The drawing under review shows one solid part. Ordinate dimensions are in mm from its lowest x, y, z. Give positions to 0.01 mm unless a question says otherwise; leave off trailing zeros. Order: outer loops, then holes, each group sorted by start corner. A loop starts at its lowest first (then second) coordinate and runs counter-clockwise, first axis right, second up. Notation, with made-up numbers: (-28, -10) -> (10, -10) arc R13 cw to (10, 8) -> close; hole circle Ø4 at (-25.5, -22). An arc over 180 degrees is marked (long way). Use a Markdown table: item, result. Add a question column.
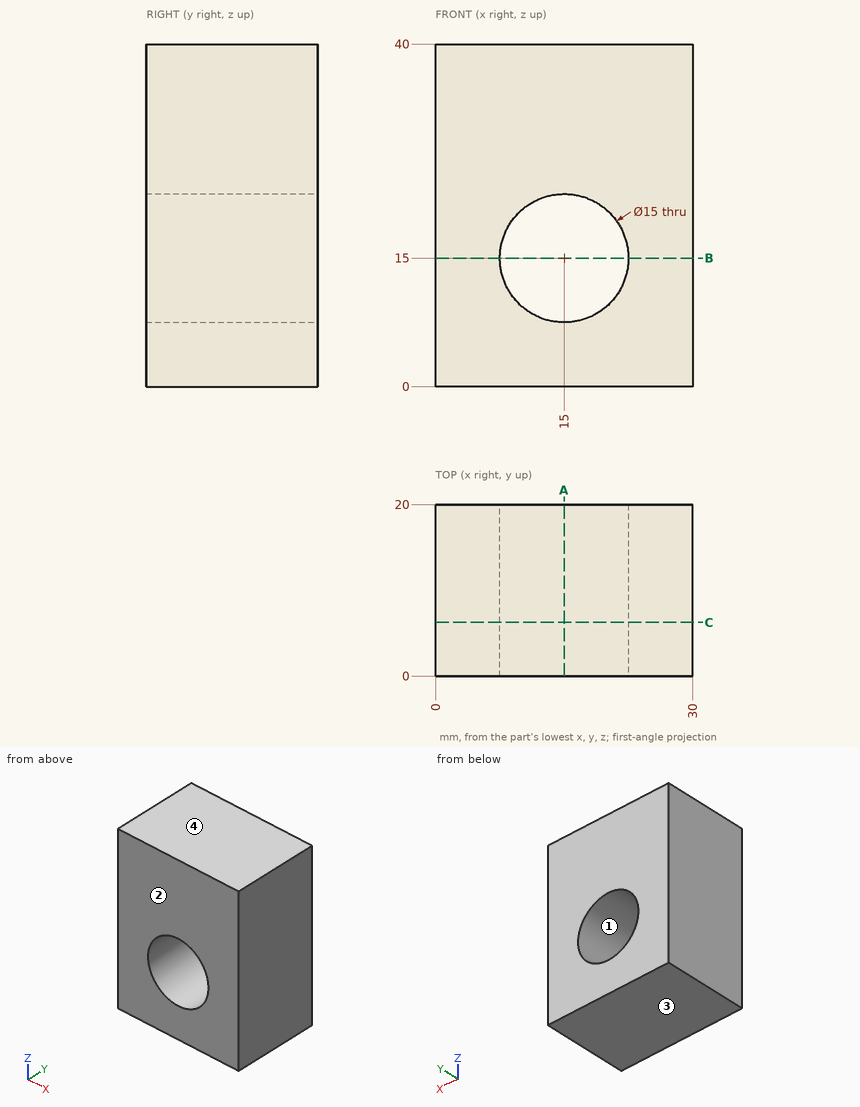
1) For L1, parallel to Z at x = 15, y = 14.5; L2, parallel to X at y = 4.75, z = 15; L3, parallel to Z at x = 16.5, y = 12.5, list the stretches that pass through material, from the lowest coordinate up. Write a range as [from, to].
2) The part is to be moulded in two halves that separate along Z. For the marked faces 1, 2, 3 and 4, say which applies: +Z half, -Z half, draft (parallel to the pull), parting line (faces both ways), or undercut.
3) Add section B-B (z = 15). Give the boundary of the cut face in (x, y).
4) Add section A-A (x = 15). Give the boundary of the cut face in (y, z).
5) Add section C-C (y = 6.25). Give the boundary of the cut face in (x, z), then the cut area to 3 significant figures.
Worked answers:
| question | item | result |
|---|---|---|
| 1 | L1 | [0, 7.5], [22.5, 40] |
| 1 | L2 | [0, 7.5], [22.5, 30] |
| 1 | L3 | [0, 7.65], [22.35, 40] |
| 2 | face 1 | undercut |
| 2 | face 2 | draft |
| 2 | face 3 | -Z half |
| 2 | face 4 | +Z half |
| 3 | outline | (0, 0) -> (7.5, 0) -> (7.5, 20) -> (0, 20) -> close; (22.5, 0) -> (30, 0) -> (30, 20) -> (22.5, 20) -> close |
| 4 | outline | (0, 0) -> (20, 0) -> (20, 7.5) -> (0, 7.5) -> close; (0, 22.5) -> (20, 22.5) -> (20, 40) -> (0, 40) -> close |
| 5 | outline | (0, 0) -> (30, 0) -> (30, 40) -> (0, 40) -> close; hole circle Ø15 at (15, 15) |
| 5 | area | 1,020 mm^2 |
